Part model, mm, in its own coordinate system. A direction names the side the tool comes from. Round coordinates to 2 decimals unless told otherwise and drop trailing zeros. Write each loop counter-clockwise with the first axis right and the second up, starting at its lowest first coordinate (ties: lowest second). Pieces come first, ordered by that corner, then holes.
```python
from build123d import *

# Parameters (mm, degrees)
SKETCH1_R               = 12
SKETCH1_R_2             = 6.5
BOSS_EXTRUDE1_DEPTH     = 20
SKETCH2_W               = 32
SKETCH2_H               = 32
SKETCH2_R               = 6.5
BOSS_EXTRUDE2_DEPTH     = 6
SKETCH3_R               = 2.25
CUT_EXTRUDE1_DEPTH      = 31.199337741
CHAMFER1_SIZE           = 4
CUT_EXTRUDE2_START      = 20
SKETCH4_W               = 2.7
SKETCH4_H               = 7.5
CUT_EXTRUDE2_DEPTH      = 10
CUT_EXTRUDE3_DEPTH      = 31.199337741
CUT_EXTRUDE3_DEPTH_BACK = 31.199337741
SKETCH5_R               = 2


with BuildPart() as part:
    # Sketch1 → Boss-Extrude1 (new body)
    with BuildSketch(Plane(origin=(0, 0, 0), x_dir=(1, 0, 0), z_dir=(0, 1, 0))):
        with Locations(Location((0, 0, 0), (0, 0, 270))):
            Circle(SKETCH1_R)
        with Locations(Location((0, 0, 0), (0, 0, 270))):
            Circle(SKETCH1_R_2, mode=Mode.SUBTRACT)
    extrude(amount=BOSS_EXTRUDE1_DEPTH)

    # Sketch2 → Boss-Extrude2 (add)
    with BuildSketch(Plane(origin=(0, 0, 0), x_dir=(1, 0, 0), z_dir=(0, 1, 0))):
        Rectangle(SKETCH2_W, SKETCH2_H)
        with Locations(Location((0, 0, 0), (0, 0, 270))):
            Circle(SKETCH2_R, mode=Mode.SUBTRACT)
    extrude(amount=BOSS_EXTRUDE2_DEPTH)

    # Sketch3 → Cut-Extrude1 (cut, through all)
    with BuildSketch(Plane(origin=(0, 0, 0), x_dir=(1, 0, 0), z_dir=(0, 1, 0))):
        with Locations(Location((-11.313708499, 11.313708499, 0), (0, 0, 270))):
            Circle(SKETCH3_R)
        with Locations(Location((-11.313708499, -11.313708499, 0), (0, 0, 270))):
            Circle(SKETCH3_R)
        with Locations(Location((11.313708499, -11.313708499, 0), (0, 0, 270))):
            Circle(SKETCH3_R)
        with Locations(Location((11.313708499, 11.313708499, 0), (0, 0, 270))):
            Circle(SKETCH3_R)
    extrude(amount=CUT_EXTRUDE1_DEPTH, mode=Mode.SUBTRACT)

    # Chamfer1
    chamfer1_edges = [part.edges().sort_by_distance(p)[0] for p in [
        (16, 3, 16),
        (16, 3, -16),
        (-16, 3, -16),
        (-16, 3, 16),
    ]]
    chamfer(chamfer1_edges, length=CHAMFER1_SIZE)

    # Sketch4 → Cut-Extrude2 (cut)
    with BuildSketch(Plane(origin=(0, 0, 0), x_dir=(1, 0, 0), z_dir=(0, 1, 0)).offset(CUT_EXTRUDE2_START)):
        with Locations((-9, 0)):
            Rectangle(SKETCH4_W, SKETCH4_H)
    cut_extrude2 = extrude(amount=-CUT_EXTRUDE2_DEPTH, mode=Mode.SUBTRACT)

    # Sketch5 → Cut-Extrude3 (cut, two sides: drawn at the far end of the back side and taken through both)
    with BuildSketch(Plane(origin=(0, 0, 0), x_dir=(0, 0, -1), z_dir=(1, 0, 0)).offset(-CUT_EXTRUDE3_DEPTH_BACK)):
        with Locations((0, 13.75)):
            Circle(SKETCH5_R)
    extrude(amount=CUT_EXTRUDE3_DEPTH + CUT_EXTRUDE3_DEPTH_BACK, mode=Mode.SUBTRACT)

    # Mirror1: Cut-Extrude2 across plane
    add(cut_extrude2.mirror(Plane(origin=(0, 0, 0), x_dir=(0, 0, 1), z_dir=(1, 0, 0))), mode=Mode.SUBTRACT)


solid = part.part
```
Q1. Drop flat-ended pins along their axis: pin 1 (5 mm diameter, centred on y = 13.75, z = 0, fed in from +X); pin 2 (5 mm diameter, centred on x = -11.31, z = 11.31, fed in from +Y); pin 3 (3 mm diameter, centred on x = -9, y = 15, fed in from -Z). Give the stop position or say it passes through.
Values follow:
pin 1: stops at x = 12
pin 2: stops at y = 6
pin 3: stops at z = -9.37
Q2. Cut at D-D on y = 15.25. Write the cut outline in (x, z).
Values follow:
outline: (-11.93, -1.32) arc R12 ccw to (11.93, -1.32) - (10.35, -1.32) - (10.35, -3.75) - (7.65, -3.75) - (7.65, -1.32) - (6.36, -1.32) arc R6.5 cw to (-6.36, -1.32) - (-7.65, -1.32) - (-7.65, -3.75) - (-10.35, -3.75) - (-10.35, -1.32) - close; (-11.93, 1.32) - (-10.35, 1.32) - (-10.35, 3.75) - (-7.65, 3.75) - (-7.65, 1.32) - (-6.36, 1.32) arc R6.5 cw to (6.36, 1.32) - (7.65, 1.32) - (7.65, 3.75) - (10.35, 3.75) - (10.35, 1.32) - (11.93, 1.32) arc R12 ccw to start
Q3. Cut at C-C on x = 0. Write the cut outline in (y, z), plus the area to 3 significant figures.
Values follow:
outline: (0, -16) - (6, -16) - (6, -12) - (20, -12) - (20, -6.5) - (0, -6.5) - close; (0, 6.5) - (20, 6.5) - (20, 12) - (6, 12) - (6, 16) - (0, 16) - close
area: 268 mm2
Q4. Which spindle directions (+Z, -Z, +X, -X, +Y, -Y) get a long thin tool onto all of the face, cutting with end or side? Do faces 1 (the flat face through (0, 3, -16)), 2 (the flat face through (9, 15, 3.75)). Say none if no direction does.
Values follow:
face 1: -Z, +X, -X, +Y, -Y
face 2: +Y
Q5. Mould opens along Z. For faces 3 (the flat face through (14, 3, -14)), 4 (the flat face through (-5, 20, 5)), 5 (the flat face through (-10.35, 16, 0)), 6 (the flat face through (14, 3, 14)) say: +Z half, -Z half, draft (parallel to the pull), parting line (faces both ways), or undercut.
Values follow:
face 3: -Z half
face 4: draft
face 5: undercut
face 6: +Z half
Q6. Cut at A-A on y = 18.75. Write the cut outline in (x, z).
Values follow:
outline: circle Ø24 at (0, 0); hole (-10.35, -3.75) - (-7.65, -3.75) - (-7.65, 3.75) - (-10.35, 3.75) - close; hole circle Ø13 at (0, 0); hole (7.65, -3.75) - (10.35, -3.75) - (10.35, 3.75) - (7.65, 3.75) - close
Q7. Cut at B-B on z = -13. Write the cut outline in (x, y), plus the area to 3 significant figures.
Values follow:
outline: (-15, 0) - (-12.8, 0) - (-12.8, 6) - (-15, 6) - close; (-9.82, 0) - (9.82, 0) - (9.82, 6) - (-9.82, 6) - close; (12.8, 0) - (15, 0) - (15, 6) - (12.8, 6) - close
area: 144 mm2
Q8. Wall check: L1, parallel to Y at x = -11, z = 0; L2, parallel to X at y = 12, z = 2; L3, parallel to X at y = 9, z = 0. Give the ranges that are in metal, low to high.
Values follow:
L1: y = 0 to 11.75, 15.75 to 20
L2: x = -11.83 to -10.35, -7.65 to -6.18, 6.18 to 7.65, 10.35 to 11.83
L3: x = -12 to -6.5, 6.5 to 12
